Autodesk Fusion 360 part; units mm, degrees
sketch "Esquisse1" plane through (0, 0, 0) normal (0, 0, 1) x (1, 0, 0)
  line L0 (-28.5, 6.5) -> (0, 6.5)
  line L1 (0, 6.5) -> (0, 0) construction
  line L2 (0, 0) -> (-35.4205, 0) construction
  line L3 (-82.5, 9.5) -> (-49.6424, 9.5)
  line L4 (-35.4205, 0) -> (-82.5, 0) construction
  line L5 (-82.5, 0) -> (-82.5, 9.5)
  arc A0 (-49.6424, 9.5) -> (-28.5, 6.5) centre (-28.5, 82.5) ccw
  line L6 (-28.5, -6.5) -> (0, -6.5)
  arc A1 (-28.5, -6.5) -> (-49.6424, -9.5) centre (-28.5, -82.5) ccw
  line L7 (-82.5, -9.5) -> (-49.6424, -9.5)
  line L8 (-82.5, 0) -> (-82.5, -9.5)
  arc A2 (49.6424, -9.5) -> (28.5, -6.5) centre (28.5, -82.5) ccw
  line L9 (28.5, -6.5) -> (0, -6.5)
  line L10 (82.5, -9.5) -> (49.6424, -9.5)
  line L11 (82.5, 0) -> (82.5, -9.5)
  line L12 (82.5, 0) -> (82.5, 9.5)
  line L13 (82.5, 9.5) -> (49.6424, 9.5)
  arc A3 (28.5, 6.5) -> (49.6424, 9.5) centre (28.5, 82.5) ccw
  line L14 (28.5, 6.5) -> (0, 6.5)
  dimension "d1" = 28.5
  dimension "d9" = 6.5
  dimension "d10" = 152
  dimension "d13" = 82.5
  dimension "d14" = 9.5
extrude "Extrusion1" add sketch "Esquisse1" along normal blind 0.28
equation "d1 = Ln / 2"
equation "Wn = Width of narrow section"
equation "Ln = Length of narrow section"
equation "Wo = Width overall, min"
equation "Lo = Length overall, min"
equation "Dg = Distance between grips"
equation "Rf = Radius of fillet"
equation "d9 = Wn / 2"
equation "d10 = Rf * 2"
equation "d13 = Lo / 2"
equation "d14 = Wo / 2"
equation "To = Thickness"
equation "d16 = To"
Check sheet for the modelled part. Datum: model origin and axes. Units: mm. Give positions to 0.01 mm unless a question says otherwise; leave off trailing zeros. Loops run counter-clockwise (first coordinate to the right, second up) from the corner with the lowest first, then second, coordinate; pieces in that order, holes last. Notation, with made-up numbers: M -24,35.25 L 2,35.25 A26 cw 2,59.25 Z; hole C 42.5,43.5 d4. An arc over 180 degrees is marked long. Return JSON: item names as keys, results as strings. Group by question number.
1. Cross-section at D-D on x = 31. Record the boundary of the cut face in (y, z).
2. Thickness scan on L1, parallel to Y at x = -7, z = 0.2; L2, parallel to Y at x = -43, z = 0.2. Record the ranges inside material, lowest first.
3. Cross-section at B-B on y = -8. Record the boundary of the cut face in (x, z) (3 decimals).
4. Cross-section at C-C on x = -20. Record the boundary of the cut face in (y, z), plus the area to 3 significant figures.
5. Cross-section at A-A on z = 0.2. Record the boundary of the cut face in (x, y), plus the area to 3 significant figures.
Return value:
{
 "1": {"outline": "M -6.54,0 L 6.54,0 L 6.54,0.28 L -6.54,0.28 Z"},
 "2": {"L1": "-6.5 to 6.5", "L2": "-7.9 to 7.9"},
 "3": {"outline": "M -82.5,0 L -43.525,0 L -43.525,0.28 L -82.5,0.28 Z; M 43.525,0 L 82.5,0 L 82.5,0.28 L 43.525,0.28 Z"},
 "4": {"outline": "M -6.5,0 L 6.5,0 L 6.5,0.28 L -6.5,0.28 Z", "area": "3.64 mm^2"},
 "5": {"outline": "M -82.5,-9.5 L -49.64,-9.5 A76 cw -28.5,-6.5 L 28.5,-6.5 A76 cw 49.64,-9.5 L 82.5,-9.5 L 82.5,9.5 L 49.64,9.5 A76 cw 28.5,6.5 L -28.5,6.5 A76 cw -49.64,9.5 L -82.5,9.5 Z", "area": "2,620 mm^2"}
}
